```python
from build123d import *

# Parameters (mm, degrees)
F0_W      = 89
F0_H      = 45
F1_DEPTH  = 5
F2_W      = 70
F2_H      = 39
F3_DEPTH  = 25
F4_W      = 85.5
F4_H      = 41.5
F5_DEPTH  = 3
F6_W      = 8
F6_H      = 8
F7_DEPTH  = 3
F8_R      = 1
F9_DEPTH  = 25
F10_DEPTH = 25
F11_W     = 2.5
F11_H     = 2
F12_DEPTH = 25
F13_W     = 89
F13_H     = 8.5
F14_DEPTH = 25


with BuildPart() as f1:
    # F0 (on Top) → F1 (new body)
    with BuildSketch(Plane.XY):
        Rectangle(F0_W, F0_H)
    extrude(amount=F1_DEPTH)

    # F2 (on Top) → F3 (cut)
    with BuildSketch(Plane.XY):
        Rectangle(F2_W, F2_H)
    extrude(amount=F3_DEPTH, mode=Mode.SUBTRACT)

    # F4 (on Top) → F5 (cut)
    with BuildSketch(Plane.XY):
        Rectangle(F4_W, F4_H)
    extrude(amount=F5_DEPTH, mode=Mode.SUBTRACT)

    # F6 (on Top) → F7 (join)
    with BuildSketch(Plane.XY):
        with Locations((-40.5, 18.5)):
            Rectangle(F6_W, F6_H)
        with Locations((-40.5, -18.5)):
            Rectangle(F6_W, F6_H)
        with Locations((40.5, 18.5)):
            Rectangle(F6_W, F6_H)
        with Locations((40.5, -18.5)):
            Rectangle(F6_W, F6_H)
    extrude(amount=F7_DEPTH)

    # F8 (on Top) → F9 (cut)
    with BuildSketch(Plane.XY):
        with BuildLine():
            ThreePointArc((41.25, 18.5), (41.618034, 18.940983), (41.75, 19.5))
            ThreePointArc((41.75, 19.5), (39.940983, 20.618034), (39.75, 18.5))
            ThreePointArc((39.75, 18.5), (40.5, 18.75), (41.25, 18.5))
        make_face()
        with BuildLine():
            ThreePointArc((41.25, 18.5), (40.5, 18.25), (39.75, 18.5))
            ThreePointArc((39.75, 18.5), (39.940983, 16.381966), (41.75, 17.5))
            ThreePointArc((41.75, 17.5), (41.618034, 18.059017), (41.25, 18.5))
        make_face()
        with BuildLine():
            ThreePointArc((-39.75, 18.5), (-39.381966, 18.940983), (-39.25, 19.5))
            ThreePointArc((-39.25, 19.5), (-41.059017, 20.618034), (-41.25, 18.5))
            ThreePointArc((-41.25, 18.5), (-40.5, 18.75), (-39.75, 18.5))
        make_face()
        with BuildLine():
            ThreePointArc((-39.75, 18.5), (-40.5, 18.25), (-41.25, 18.5))
            ThreePointArc((-41.25, 18.5), (-41.059017, 16.381966), (-39.25, 17.5))
            ThreePointArc((-39.25, 17.5), (-39.381966, 18.059017), (-39.75, 18.5))
        make_face()
        with Locations((-39, 0)):
            Circle(F8_R)
        with Locations((39, 0)):
            Circle(F8_R)
    extrude(amount=F9_DEPTH, mode=Mode.SUBTRACT)

    # F8 (on Top) → F10 (cut)
    with BuildSketch(Plane.XY):
        with BuildLine():
            ThreePointArc((41.25, 18.5), (41.618034, 18.940983), (41.75, 19.5))
            ThreePointArc((41.75, 19.5), (39.940983, 20.618034), (39.75, 18.5))
            ThreePointArc((39.75, 18.5), (40.5, 18.75), (41.25, 18.5))
        make_face()
        with BuildLine():
            ThreePointArc((41.25, 18.5), (40.5, 18.25), (39.75, 18.5))
            ThreePointArc((39.75, 18.5), (39.940983, 16.381966), (41.75, 17.5))
            ThreePointArc((41.75, 17.5), (41.618034, 18.059017), (41.25, 18.5))
        make_face()
        with BuildLine():
            ThreePointArc((-39.75, 18.5), (-39.381966, 18.940983), (-39.25, 19.5))
            ThreePointArc((-39.25, 19.5), (-41.059017, 20.618034), (-41.25, 18.5))
            ThreePointArc((-41.25, 18.5), (-40.5, 18.75), (-39.75, 18.5))
        make_face()
        with BuildLine():
            ThreePointArc((-39.75, 18.5), (-40.5, 18.25), (-41.25, 18.5))
            ThreePointArc((-41.25, 18.5), (-41.059017, 16.381966), (-39.25, 17.5))
            ThreePointArc((-39.25, 17.5), (-39.381966, 18.059017), (-39.75, 18.5))
        make_face()
        with Locations((-39, 0)):
            Circle(F8_R)
        with Locations((39, 0)):
            Circle(F8_R)
    extrude(amount=F10_DEPTH, mode=Mode.SUBTRACT)

    # F11 (on face) → F12 (cut)
    with BuildSketch(Plane(origin=(0, 0, 0), x_dir=(1, 0, 0), z_dir=(0, 0, -1))):
        with Locations((-40.5, -18.5)):
            Rectangle(F11_W, F11_H)
        with Locations((40.5, -18.5)):
            Rectangle(F11_W, F11_H)
    extrude(amount=-F12_DEPTH, mode=Mode.SUBTRACT)

    # F13 (on face) → F14 (cut)
    with BuildSketch(Plane.XY.offset(5)):
        with Locations((0, -18.25)):
            Rectangle(F13_W, F13_H)
    extrude(amount=-F14_DEPTH, mode=Mode.SUBTRACT)


solid = f1.part
```
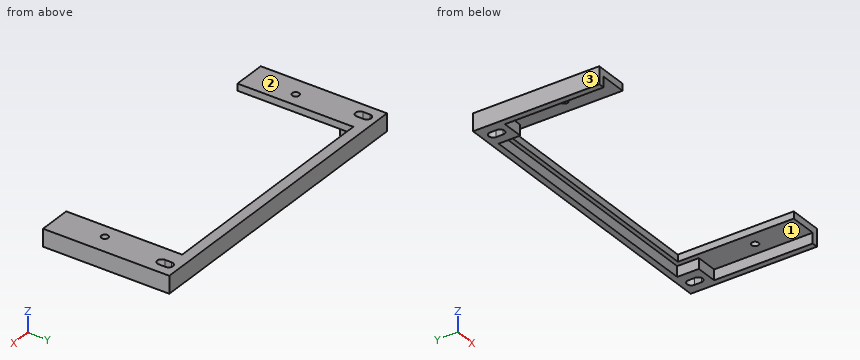
For this review, take the finished solid that the model builds, in its own axes (mm). Face numbers are marked on the shaded views. Give positions to 0.01 mm unless a question says otherwise; leave off trailing zeros. Loops run counter-clockwise (first coordinate to the right, second up) from the corner with the lowest first, then second, coordinate; pieces in that order, holes last. Notation, with made-up numbers: M 7,3 L 32,3 A21 ccw 32,15 Z; hole C 25.25,-37 d1. An arc over 180 degrees is marked long. One line per item, written item: value. Start each with the question number.
Q1. Draft analysis for pull direction X (two halves, no side actions). For the marked faces 1, 2 and 3, state which applies: released by +X, released by -X, zero draft, split by the parting line, or undercut.
Q2. Add section D-D (x = 27). Give the boundary of the cut face in (y, z), and give its area (4 significant figures).
Q3. Add section A-A (y = 4). Give the boundary of the cut face in (x, z).
Q4. Clearance check with flat-ended pins moving along their axes: pin 1 Ø2 at (x, z) = (-8, 4) entering from -Y; pin 2 Ø1.5 at (x, z) = (15.5, 0.5) entering from -Y. State where each tip first meets the part, or that it passes through.
Q5. Add section C-C (y = 0). Give the boundary of the cut face in (x, z), and give its area (3 significant figures).
Q6. For L1, parallel to X at y = 0, z = 3.4; L2, parallel to X at y = 20.5, z = 3.85; L3, parallel to X at y = -0.5, z = 2.75, list the stretches that pass through material, from the lowest coordinate up.
Q7. Add section B-B (z = 1.95). Give the boundary of the cut face in (x, y), and give its area (3 significant figures).
Reply:
1. face 1: undercut
1. face 2: zero draft
1. face 3: released by -X
2. outline: M 19.5,3 L 20.75,3 L 20.75,0 L 22.5,0 L 22.5,5 L 19.5,5 Z
2. area: 11.25 mm²
3. outline: M -44.5,0 L -42.75,0 L -42.75,3 L -35,3 L -35,5 L -44.5,5 Z; M 35,3 L 42.75,3 L 42.75,0 L 44.5,0 L 44.5,5 L 35,5 Z
4. pin 1: y = 19.5
4. pin 2: y = 20.75
5. outline: M -44.5,0 L -42.75,0 L -42.75,3 L -40,3 L -40,5 L -44.5,5 Z; M -38,3 L -35,3 L -35,5 L -38,5 Z; M 35,3 L 38,3 L 38,5 L 35,5 Z; M 40,3 L 42.75,3 L 42.75,0 L 44.5,0 L 44.5,5 L 40,5 Z
5. area: 40.5 mm²
6. L1: -44.5 to -40, -38 to -35, 35 to 38, 40 to 44.5
6. L2: -44.5 to -41.25, -39.75 to 39.75, 41.25 to 44.5
6. L3: -44.5 to -42.75, 42.75 to 44.5
7. outline: M -44.5,-14 L -42.75,-14 L -42.75,14.5 L -36.5,14.5 L -36.5,20.75 L 36.5,20.75 L 36.5,14.5 L 42.75,14.5 L 42.75,-14 L 44.5,-14 L 44.5,22.5 L -44.5,22.5 Z; hole M -41.75,17.5 A1.25 ccw -39.25,17.5 L -39.25,19.5 A1.25 ccw -41.75,19.5 Z; hole M 39.25,17.5 A1.25 ccw 41.75,17.5 L 41.75,19.5 A1.25 ccw 39.25,19.5 Z
7. area: 336 mm²
